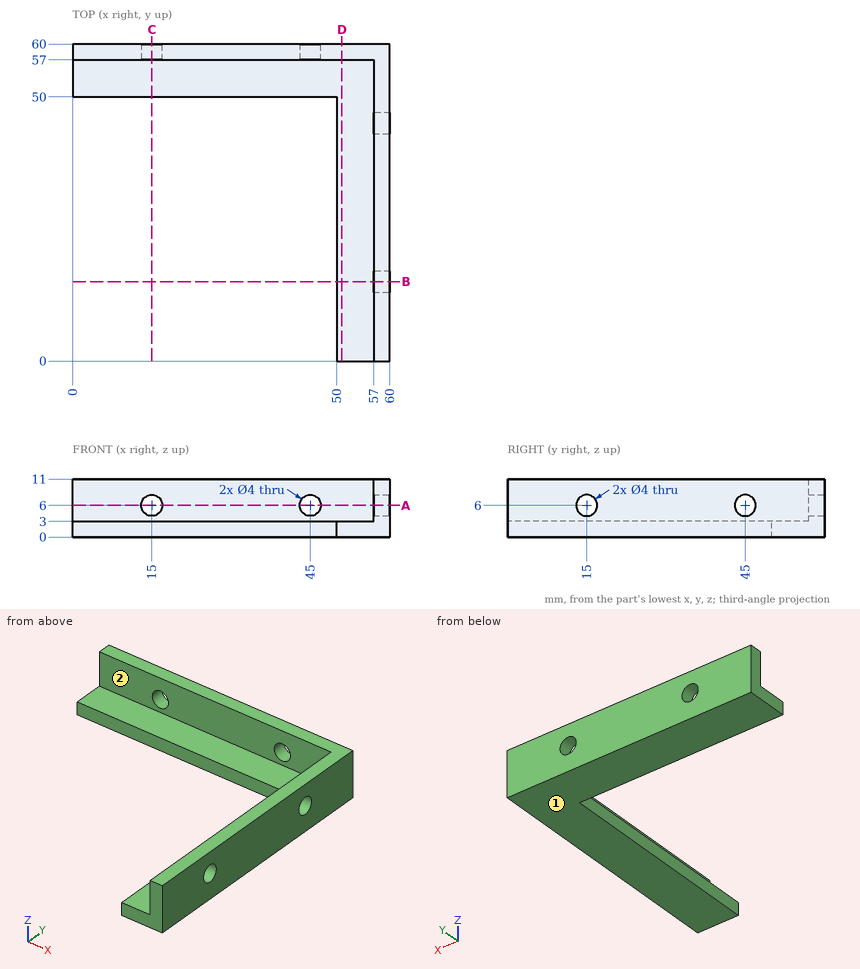
Source: three-view drawing plus pictorial views. Frame: mm from the lowest corner of the part. A direction names the side the tool comes from. Round coordinates to 2 decimals unless told otherwise and drop trailing zeros. Write each loop counter-clockwise with the first axis right and the second up, starting at its lowest first coordinate (ties: lowest second). Pieces come first, ordered by that corner, then holes. Notation, with made-up numbers: (-24, -6) -> (-20, -6) arc R16 cw to (-20, 24) -> close; hole circle Ø2 at (-23, -16). An arc over 180 degrees is marked (long way). Return JSON: item names as keys, results as strings.
Q1. Section D-D on x = 51. Return the cut outline in (y, z).
From the geometry:
{"outline": "(0, 0) -> (60, 0) -> (60, 11) -> (57, 11) -> (57, 3) -> (0, 3) -> close"}
Q2. Section A-A on z = 6. Return the cut outline in (x, y), and give its area (3 significant figures).
From the geometry:
{"outline": "(0, 57) -> (13, 57) -> (13, 60) -> (0, 60) -> close; (17, 57) -> (43, 57) -> (43, 60) -> (17, 60) -> close; (47, 57) -> (57, 57) -> (57, 47) -> (60, 47) -> (60, 60) -> (47, 60) -> close; (57, 0) -> (60, 0) -> (60, 13) -> (57, 13) -> close; (57, 17) -> (60, 17) -> (60, 43) -> (57, 43) -> close", "area": "303 mm2"}
Q3. First-contact query: pin 1 Ø4 at (x, y) = (53.5, 44.5) entering from -Z; pin 2 Ø2 at (x, z) = (19, 7.5) entering from -Y; pin 3 Ø1.5 at (x, z) = (32, 1.5) entering from -Y; pin 4 Ø6.5 at (y, z) = (36.5, 8.5) entering from -X. Flat tips, straight axial feed; report the tip coordinate or a pass-through.
From the geometry:
{"pin 1": "z = 0", "pin 2": "y = 57", "pin 3": "y = 50", "pin 4": "x = 57"}
Q4. Section B-B on y = 15. Return the cut outline in (x, z), and give its area (3 significant figures).
From the geometry:
{"outline": "(50, 0) -> (60, 0) -> (60, 4) -> (57, 4) -> (57, 3) -> (50, 3) -> close; (57, 8) -> (60, 8) -> (60, 11) -> (57, 11) -> close", "area": "42.0 mm2"}
Q5. Set-up query: the marked faces 1 and 2. Return all of +Z, -Z, +X, -X, +Y, -Y with unobstructed straight access to the full face (end or side cutting, diameter ignored); none if empty.
From the geometry:
{"face 1": "-Z, +X, -X, +Y, -Y", "face 2": "+Z, -X, -Y"}
Q6. Ray query, line 1 (Z direction, x = 58.45, y = 15); line 2 (Y direction, x = 24, z = 3.75). Return the intervals inside material, ascending.
From the geometry:
{"line 1": "0 to 4, 8 to 11", "line 2": "57 to 60"}
